```python
from build123d import *

# Parameters (mm, degrees)
F0_R      = 75
F1_DEPTH  = 5
F0_R_2    = 79
F2_DEPTH  = 30
F3_R      = 142.5
F3_R_2    = 79
F3_R_3    = 75
F4_DEPTH  = 5
F3_R_4    = 145.5
F5_DEPTH  = 158
F6_DEPTH  = 180
F7_R      = 150.5
F7_R_2    = 145.5
F7_R_3    = 142.5
F8_DEPTH  = 7.5
F9_R      = 150.5
F9_R_2    = 147
F10_DEPTH = 13
F11_R     = 7
F11_R_2   = 4
F12_DEPTH = 7
F13_D     = 5.5
F13_DEPTH = 12
F13_TIP   = 1.6523667023


with BuildPart() as f1:
    # F0 (on Top) → F1 (new body)
    with BuildSketch(Plane.XY):
        Circle(F0_R)
        with BuildLine():
            ThreePointArc((-27.2772727273, 3.4929060339), (0, 27.5), (27.2772727273, 3.4929060339))
            ThreePointArc((27.2772727273, 3.4929060339), (31, 0), (27.2772727273, -3.4929060339))
            ThreePointArc((27.2772727273, -3.4929060339), (0, -27.5), (-27.2772727273, -3.4929060339))
            ThreePointArc((-27.2772727273, -3.4929060339), (-31, 0), (-27.2772727273, 3.4929060339))
        make_face(mode=Mode.SUBTRACT)
    extrude(amount=F1_DEPTH)

    # F0 (on Top) → F2 (join)
    with BuildSketch(Plane.XY):
        Circle(F0_R_2)
        Circle(F0_R, mode=Mode.SUBTRACT)
    extrude(amount=F2_DEPTH)

    # F3 (on face) → F4 (join)
    with BuildSketch(Plane.XY.offset(30)):
        Circle(F3_R)
        Circle(F3_R_2, mode=Mode.SUBTRACT)
        Circle(F3_R_2)
        Circle(F3_R_3, mode=Mode.SUBTRACT)
    extrude(amount=F4_DEPTH)

    # F3 (on face) → F5 (join)
    with BuildSketch(Plane.XY.offset(30)):
        Circle(F3_R_4)
        Circle(F3_R, mode=Mode.SUBTRACT)
    extrude(amount=F5_DEPTH)

    # F3 (on face) → F6 (join)
    with BuildSketch(Plane.XY.offset(30)):
        Circle(F3_R_4)
        Circle(F3_R, mode=Mode.SUBTRACT)
    extrude(amount=-F6_DEPTH)

    # F7 (on face) → F8 (join)
    with BuildSketch(Plane(origin=(0, 0, -150), x_dir=(1, 0, 0), z_dir=(0, 0, -1))):
        Circle(F7_R)
        Circle(F7_R_2, mode=Mode.SUBTRACT)
        Circle(F7_R_2)
        Circle(F7_R_3, mode=Mode.SUBTRACT)
    extrude(amount=F8_DEPTH)

    # F9 (on face) → F10 (join)
    with BuildSketch(Plane(origin=(0, 0, -157.5), x_dir=(1, 0, 0), z_dir=(0, 0, -1))):
        Circle(F9_R)
        Circle(F9_R_2, mode=Mode.SUBTRACT)
    extrude(amount=F10_DEPTH)

    # F11 (on face) → F12 (join)
    with BuildSketch(Plane.XY.offset(35)):
        with Locations((0, 83.2192561637)):
            Circle(F11_R)
        with Locations((0, 83.2192561637)):
            Circle(F11_R_2, mode=Mode.SUBTRACT)
        with Locations((-65, -51.9658021822)):
            Circle(F11_R)
        with Locations((-65, -51.9658021822)):
            Circle(F11_R_2, mode=Mode.SUBTRACT)
        with Locations((65, -51.9658021822)):
            Circle(F11_R)
        with Locations((65, -51.9658021822)):
            Circle(F11_R_2, mode=Mode.SUBTRACT)
    extrude(amount=F12_DEPTH)

    # F13
    with Locations(Plane.XY.offset(35)):
        with Locations((0, 83.2192561637), (-65, -51.9658021822), (65, -51.9658021822)):
            Hole(F13_D / 2, depth=F13_DEPTH)
            with Locations((0, 0, -(F13_DEPTH + F13_TIP / 2))):  # 118° drill point
                Cone(0, F13_D / 2, F13_TIP, mode=Mode.SUBTRACT)


solid = f1.part
```
Verification items for the finished model (mm, model axes). A direction names the side the tool comes from. Give positions to 0.01 mm unless a question says otherwise; leave off trailing zeros. Loops run counter-clockwise (first coordinate to the right, second up) from the corner with the lowest first, then second, coordinate; pieces in that order, holes last. Notation, with made-up numbers: M -21,-17 L 13,-17 A26 ccw 13,-1 Z; hole C 69,-4.75 d8. An arc over 180 degrees is marked long. Return JSON: item names as keys, results as strings.
1) Gauge pin test, flat ends, axial feed: P1, Ø9, axis at x = 1, y = 82, coming from the +Z side; P2, Ø7, axis at x = -65, y = -51.97, coming from the +Z side; P3, Ø7, axis at x = 0, y = 83.22, coming from the -Z side. Record the tip position at first contact, or that the pin passes through.
Findings:
{"P1": "stops at z = 42", "P2": "stops at z = 35", "P3": "stops at z = 30"}
2) Section check C-C, the plane z = -18.5. Enter the section's corners in (x, y), and give its area (3 significant figures).
Findings:
{"outline": "C 0,0 d291; hole C 0,0 d285", "area": "2,710 mm2"}
3) Mould release check, pull along X, two halves, no side actions. Record for faces 5 (the flat face through (33, 144, -170.5)), 6 (the cylindrical face through (138.781, 43.704, 21.366)), 7 (the cylindrical face through (-1.517, 76.386, 38.451)): released by +X, released by -X, zero draft, split by the parting line, or undercut.
Findings:
{"face 5": "zero draft", "face 6": "split by the parting line", "face 7": "undercut"}
4) Section check B-B, the plane y = 117. Enter the section's corners in (x, z).
Findings:
{"outline": "M -94.66,-170.5 L -88.99,-170.5 L -88.99,-157.5 L -81.35,-157.5 L -81.35,30 L 81.35,30 L 81.35,-157.5 L 88.99,-157.5 L 88.99,-170.5 L 94.66,-170.5 L 94.66,-150 L 86.49,-150 L 86.49,188 L 81.35,188 L 81.35,35 L -81.35,35 L -81.35,188 L -86.49,188 L -86.49,-150 L -94.66,-150 Z"}
5) Material ranges on L1, parallel to X at y = 0, z = -152.5; L2, parallel to Y at x = 65, z = 32.95; L3, parallel to Y at x = -2, z = -98, recorded low to high. Write a range as [from, to].
Findings:
{"L1": "x = [-150.5, -142.5], [142.5, 150.5]", "L2": "y = [-130.17, -54.72], [-49.22, -37.42], [37.42, 130.17]", "L3": "y = [-145.49, -142.49], [142.49, 145.49]"}
6) Tool access check on faces 1 (the flat face through (-79, -123, -150)), 2 (the cylindrical face through (-0.556, 27.494, 2.465)), 3 (the flat face through (107, -96, 188)), 4 (the flat face through (-76.9, -120.5, -157.5)). Record the directions out of +Z, -Z, +X, -X, +Y, -Y that give a thin tool (end or side, any length) a straight path to the whole face; none if there is none.
Findings:
{"face 1": "+Z", "face 2": "+Z, -Z", "face 3": "+Z, +X, -X, +Y, -Y", "face 4": "-Z"}
7) Section check A-A, the plane x = -36.5. Enter the section's corners in (y, z), and give its area (3 significant figures).
Findings:
{"outline": "M -146.01,-170.5 L -142.4,-170.5 L -142.4,-157.5 L -137.75,-157.5 L -137.75,30 L -70.06,30 L -70.06,0 L 70.06,0 L 70.06,30 L 137.75,30 L 137.75,-157.5 L 142.4,-157.5 L 142.4,-170.5 L 146.01,-170.5 L 146.01,-150 L 140.85,-150 L 140.85,188 L 137.75,188 L 137.75,35 L 65.52,35 L 65.52,5 L -65.52,5 L -65.52,35 L -137.75,35 L -137.75,188 L -140.85,188 L -140.85,-150 L -146.01,-150 Z", "area": "3,960 mm2"}
